Geometry: final body of the model. Coordinates: model frame, mm. A direction names the side the tool comes from. Coordinates: 2 decimals unless noted, no trailing zeros. Write each loop counter-clockwise with the first axis right and the second up, starting at its lowest first coordinate (ties: lowest second). Pieces come first, ordered by that corner, then holes. Notation, with made-up numbers: (-22.5, 14) - (8.5, 14) arc R17 cw to (8.5, 25) - close; hole circle Ø11 at (59.5, 23). An arc over 180 degrees is marked (long way). Answer as a JSON object with one key per item and string values. Group by question number.
Item 1: Mould query, pull axis Z, two halves, no side actions, for faces 4 (the cylindrical face through (-12.665, 6.887, 57.377)), 5 (the flat face through (-14, 0, -2)), 6 (the cylindrical face through (-14.6, 85.88, 27.67)). Classes: pulls with the +Z half, pulls with the -Z half, needs draft (parallel to the pull), parting line crosses it, or undercut.
Item 2: Section A-A on z = 15.5. Return loops of the section in (x, y), and give its area (3 significant figures).
Item 3: Line query: line 1 along Y through (x, z) = (-11, 19.5); line 2 along X through (y, z) = (80, 13); line 3 along Z through (x, y) = (-11.5, 22.5). Output: solid intervals per line, ascending. Write a range as from..to.
Item 4: First-contact query: pin 1 Ø3 at (x, y) = (5.5, 46.5) entering from +Z; pin 2 Ø10 at (x, y) = (-6.5, 46.5) entering from -Z; pin 3 Ø1 at (y, z) = (46, -40.5) entering from +X; pin 4 Ø8 at (x, z) = (-13.18, 34.06) entering from -Y. Flat tips, straight axial feed; report the tip coordinate or a pass-through.
Item 5: Section D-D on x = -15. Return loops of the section in (y, z), and give its area (3 significant figures).
Item 6: Section B-B on x = -32. Return loops of the section in (y, z).
Item 7: Set-up query: faces 1 (the cylindrical face through (-13.824, 86.073, 57.636)), 2 (the cylindrical face through (-18.36, 45.71, -61.86)), 3 (the flat face through (9.843, 86, -1)). Return all of +Z, -Z, +X, -X, +Y, -Y with unobstructed straight access to the full face (end or side cutting, diameter ignored); none if empty.
Item 8: Section C-C on z = 31. Return loops of the section in (x, y).
```python
from build123d import *

# Parameters (mm, degrees)
F0_R      = 23.1868953792
F1_DEPTH  = 92.71
F3_DEPTH  = 13.97
F5_DEPTH  = 13.97
F7_DEPTH  = 13.462
F9_DEPTH  = 13.462
F10_R     = 7.1263406122
F11_DEPTH = 92.711
F12_R     = 6.5437745526
F13_DEPTH = 92.711


with BuildPart() as f1:
    # F0 (on Front) → F1 (new body)
    with BuildSketch(Plane.XZ):
        with Locations((-13.3315408602, -39.2239503562)):
            Circle(F0_R)
    extrude(amount=-F1_DEPTH)

    # F2 (on face) → F3 (join)
    with BuildSketch(Plane.XZ):
        with BuildLine():
            Line((-36.5160371978, 34.0590924025), (-36.5160371978, -38.8904134022))
            ThreePointArc((-36.5160371978, -38.8904134022), (-13.3315408602, -16.0370549771), (9.8529554773, -38.8904134022))
            Line((9.8529554773, -38.8904134022), (10.1600009948, -38.8904134022))
            Line((10.1600009948, -38.8904134022), (10.1600009948, 34.0590924025))
            Line((10.1600009948, 34.0590924025), (-36.5160371978, 34.0590924025))
        make_face()
    extrude(amount=-F3_DEPTH)

    # F4 (on face) → F5 (join)
    with BuildSketch(Plane.XZ):
        with BuildLine():
            Line((-36.5011457602, 34.0590924025), (10.1451095572, 34.0590924025))
            ThreePointArc((10.1451095572, 34.0590924025), (-13.1780181015, 57.3822200612), (-36.5011457602, 34.0590924025))
        make_face()
    extrude(amount=-F5_DEPTH)

    # F6 (on face) → F7 (join)
    with BuildSketch(Plane(origin=(0, 92.71, 0), x_dir=(-1, 0, 0), z_dir=(0, 1, 0))):
        with BuildLine():
            Line((-9.8427801074, 34.751817584), (-9.8427801074, -38.4604289001))
            ThreePointArc((-9.8427801074, -38.4604289001), (13.0780994515, -16.038440123), (36.4836342633, -37.954033673))
            Line((36.4836342633, -37.954033673), (36.4836342633, 34.751817584))
            Line((36.4836342633, 34.751817584), (-9.8427801074, 34.751817584))
        make_face()
    extrude(amount=-F7_DEPTH)

    # F8 (on face) → F9 (join)
    with BuildSketch(Plane(origin=(0, 92.71, 0), x_dir=(-1, 0, 0), z_dir=(0, 1, 0))):
        with BuildLine():
            Line((-9.5691616246, 34.751817584), (36.2100157805, 34.751817584))
            ThreePointArc((36.2100157805, 34.751817584), (13.3204270779, 57.6414062866), (-9.5691616246, 34.751817584))
        make_face()
    extrude(amount=-F9_DEPTH)

    # F10 (on face) → F11 (cut, through all)
    with BuildSketch(Plane.XZ):
        with Locations((-13.3315408602, -39.2239503562)):
            Circle(F10_R)
    extrude(amount=-F11_DEPTH, mode=Mode.SUBTRACT)

    # F12 (on face) → F13 (cut, through all)
    with BuildSketch(Plane.XZ):
        with Locations((-13.1780181015, 34.0590924025)):
            Circle(F12_R)
    extrude(amount=-F13_DEPTH, mode=Mode.SUBTRACT)


solid = f1.part
```
Checks:
{
 "1": {"face 4": "pulls with the +Z half", "face 5": "needs draft", "face 6": "undercut"},
 "2": {"outline": "(-36.52, 0) - (10.16, 0) - (10.16, 13.97) - (-36.52, 13.97) - close; (-36.48, 79.25) - (9.84, 79.25) - (9.84, 92.71) - (-36.48, 92.71) - close", "area": "1,280 mm^2"},
 "3": {"line 1": "0..13.97, 79.25..92.71", "line 2": "-36.48..9.84", "line 3": "-62.34..-46.11, -32.34..-16.11"},
 "4": {"pin 1": "z = -23.82", "pin 2": "z = -62.34", "pin 3": "x = 9.84", "pin 4": "through"},
 "5": {"outline": "(0, -62.35) - (92.71, -62.35) - (92.71, -46.15) - (0, -46.15) - close; (0, -32.3) - (92.71, -32.3) - (92.71, 27.77) - (79.25, 27.77) - (79.25, -16.1) - (13.97, -16.1) - (13.97, 27.77) - (0, 27.77) - close; (0, 40.34) - (13.97, 40.34) - (13.97, 57.31) - (0, 57.31) - close; (79.25, 40.34) - (92.71, 40.34) - (92.71, 57.58) - (79.25, 57.58) - close", "area": "4,680 mm^2"},
 "6": {"outline": "(0, -52.98) - (92.71, -52.98) - (92.71, 47.98) - (79.25, 47.98) - (79.25, -25.47) - (13.97, -25.47) - (13.97, 47.83) - (0, 47.83) - close"},
 "7": {"face 1": "+Z, +Y", "face 2": "none", "face 3": "+Z, -Z, +X, +Y"},
 "8": {"outline": "(-36.52, 0) - (-18.96, 0) - (-18.96, 13.97) - (-36.52, 13.97) - close; (-36.48, 79.25) - (-18.96, 79.25) - (-18.96, 92.71) - (-36.48, 92.71) - close; (-7.39, 0) - (10.16, 0) - (10.16, 13.97) - (-7.39, 13.97) - close; (-7.39, 79.25) - (9.84, 79.25) - (9.84, 92.71) - (-7.39, 92.71) - close"}
}
